Autodesk Inventor part; units mm, degrees
ref_plane "YZ Plane" through (0, 0, 0) normal (1, 0, 0) x (0, 1, 0)
ref_plane "XZ Plane" through (0, 0, 0) normal (0, 1, 0) x (-1, 0, 0)
ref_plane "XY Plane" through (0, 0, 0) normal (0, 0, 1) x (1, 0, 0)
sketch "Sketch1" plane through (0, 0, 0) normal (0, 1, 0) x (-1, 0, 0)
  line L0 (45, 192.5) -> (-45, 192.5)
  line L1 (-45, 192.5) -> (-45, -192.5)
  line L2 (-45, -192.5) -> (45, -192.5)
  line L3 (45, -192.5) -> (45, 192.5)
  line L4 (45, 192.5) -> (-45, -192.5) construction
  line L5 (-45, 192.5) -> (45, -192.5) construction
  line L6 (45, 138.0648) -> (24, 138.0648)
  line L7 (24, 138.0648) -> (24, 113.0648)
  line L8 (24, 113.0648) -> (-11, 113.0648)
  line L9 (-11, 113.0648) -> (-11, 62.0648)
  line L10 (-11, 62.0648) -> (-15.9497, 57.115)
  line L11 (-15.9497, 57.115) -> (-15.9497, -142.885)
  line L12 (-15.9497, -142.885) -> (25.0503, -142.885)
  line L13 (25.0503, -142.885) -> (24, -192.5)
  line L14 (-45, 151.0874) -> (10, 151.0874)
  line L15 (10, 151.0874) -> (10, 180.0874)
  line L16 (10, 180.0874) -> (45, 180.0874)
  line L17 (10, 192.5) -> (-0.6066, 181.8934)
  line L18 (-0.6066, 181.8934) -> (-0.6066, 161.8934)
  line L19 (-0.6066, 161.8934) -> (-35.6066, 161.8934)
  line L20 (-35.6066, 161.8934) -> (-46.4126, 151.0874)
  line L21 (-0.6066, 161.8934) -> (10, 151.0874)
  line L22 (10, 180.0874) -> (3.7937, 186.2937)
  point P0 (0, 0)
  point P1 (-45, 152.5)
  dimension "d0" = 90
  dimension "d1" = 385
  dimension "d25" = 21
  dimension "d27" = 25
  dimension "d28" = 35
  dimension "d29" = 51
  dimension "d30" = 7
  dimension "d31" = 135
  dimension "d32" = 200
  dimension "d33" = 41
  dimension "d34" = 55
  dimension "d35" = 29
  dimension "d36" = 15
  dimension "d37" = 20
  dimension "d38" = 35
extrude "Extrusion1" add sketch "Sketch1" along normal blind 70 contours L3 L16 L22 L17 L0 | L3 L6 L7 L8 L9 L10 L11 L12 L13 L2 L1 L14 L15 L16 | L22 L15 L21 L18 L17 | L20 L19 L21 L14 L1
fillet "Fillet1" radius 20 1 edges at (45, 35, -192.5)
sketch "Sketch2" plane through (0, 70, 0) normal (0, 1, 0) x (1, 0, 0)
  arc A0 (45, 172.5) -> (25, 192.5) centre (25, 172.5) ccw
  line L0 (45, 172.5) -> (25, 172.5)
  line L1 (25, 172.5) -> (25, -161.8934)
  line L2 (0.6066, -161.8934) -> (35.6066, -161.8934)
  line L3 (25, 172.5) -> (25, 192.5171)
  line L4 (25, 192.5171) -> (25, 80.0171)
  line L5 (25, 80.0171) -> (15.9497, 80.0171)
  line L6 (15.9497, 142.885) -> (15.9497, -57.115)
  line L7 (25, 80.0171) -> (25, 5.0171)
  line L8 (25, 5.0171) -> (15.9497, 5.0171)
  line L9 (15.9497, 80.0171) -> (15.9497, 5.0171)
  arc A1 (45, 172.5) -> (25, 192.5) centre (25, 172.5) ccw
  line L10 (25, 192.5) -> (-24, 192.5)
  line L11 (-24, 192.5) -> (-25.0503, 142.885)
  line L12 (-25.0503, 142.885) -> (15.9497, 142.885)
  line L13 (15.9497, 142.885) -> (15.9497, -57.115)
  line L14 (15.9497, -57.115) -> (11, -62.0648)
  line L15 (11, -62.0648) -> (11, -113.0648)
  line L16 (11, -113.0648) -> (-24, -113.0648)
  line L17 (-24, -113.0648) -> (-24, -138.0648)
  line L18 (-24, -138.0648) -> (-45, -138.0648)
  line L19 (-45, -138.0648) -> (-45, -192.5)
  line L20 (45, -152.5) -> (45, 172.5)
  line L21 (25, 5.0171) -> (25, -127.4829)
  line L22 (25, -127.4829) -> (-24, -127.4829)
  line L23 (-45, -192.5) -> (-10, -192.5)
  line L24 (-10, -192.5) -> (0.6066, -181.8934)
  line L25 (0.6066, -181.8934) -> (0.6066, -161.8934)
  line L26 (0.6066, -161.8934) -> (35.6066, -161.8934)
  line L27 (35.6066, -161.8934) -> (45, -152.5)
  point P0 (0, 0)
  dimension "d45" = 112.5
  dimension "d46" = 75
  dimension "d47" = 132.5
extrude "Extrusion2" cut sketch "Sketch2" against normal blind 4 contours L3 L1 L5 L6 L12 L11 L10 | L1 L22 L17 L16 L15 L14 L6 L8
sketch "Sketch3" plane through (0, 0, 0) normal (0, -1, 0) x (1, 0, 0)
  line L0 (25, -192.5) -> (25, -80.0171)
  line L1 (25, -80.0171) -> (15.9497, -80.0171)
  line L2 (15.9497, -5.0171) -> (25, -5.0171)
  line L3 (25, -5.0171) -> (25, 127.4829)
  line L4 (25, 127.4829) -> (-24, 127.4829)
  arc A0 (25, -192.5) -> (45, -172.5) centre (25, -172.5) ccw
  line L5 (45, 152.5) -> (45, -172.5)
  line L6 (35.6066, 161.8934) -> (45, 152.5)
  line L7 (0.6066, 161.8934) -> (35.6066, 161.8934)
  line L8 (0.6066, 181.8934) -> (0.6066, 161.8934)
  line L9 (-10, 192.5) -> (0.6066, 181.8934)
  line L10 (-45, 192.5) -> (-10, 192.5)
  line L11 (-45, 138.0648) -> (-45, 192.5)
  line L12 (-24, 138.0648) -> (-45, 138.0648)
  line L13 (-24, 113.0648) -> (-24, 138.0648)
  line L14 (11, 113.0648) -> (-24, 113.0648)
  line L15 (11, 62.0648) -> (11, 113.0648)
  line L16 (15.9497, 57.115) -> (11, 62.0648)
  line L17 (15.9497, -142.885) -> (15.9497, 57.115)
  line L18 (-25.0503, -142.885) -> (15.9497, -142.885)
  line L19 (-24, -192.5) -> (-25.0503, -142.885)
  line L20 (25, -192.5) -> (-24, -192.5)
  point P0 (0, 0)
extrude "Extrusion3" cut sketch "Sketch3" against normal blind 4 contours L20 L19 L18 L17 L1 L0 | L17 L16 L15 L14 L13 L4 L3 L2
chamfer "Chamfer2" distance 9.3934 angle 45 1 edges at (18.1066, 70, 161.8934)
chamfer "Chamfer3" distance 9.3934 angle 45 2 edges at (0.6066, 70, 171.8934) (-27.5, 70, 192.5)
chamfer "Chamfer4" distance 9.3934 angle 45 1 edges at (18.1066, 0, 161.8934)
chamfer "Chamfer5" distance 9.3934 angle 45 2 edges at (0.6066, 0, 171.8934) (-27.5, 0, 192.5)
sketch "Sketch4" plane through (-45, 0, 138.0648) normal (-1, 0, 0) x (0, 0, 1)
  line L0 (0, 0) -> (0, 70)
  line L1 (0, 0) -> (54.4352, 70)
  line L2 (0, 70) -> (54.4352, 0)
  circle A0 centre (27.2176, 35) radius 18.5
  point P0 (-138.0648, 0)
  dimension "d64" = 37
extrude "Extrusion4" cut sketch "Sketch4" against normal blind 39 contours A0 L2 L1 | L1 L2 A0 | A0 L1 L2 | L1 A0 L2
Can you work these out from the model? Positions are in its coordinate system, mm. A direction names the side the tool comes from. Coordinates: 2 decimals unless noted, no trailing zeros. Loops run counter-clockwise (first coordinate to the right, second up) from the corner with the lowest first, then second, coordinate; pieces in that order, holes last. Notation, with made-up numbers: (1, 43.25) - (46, 43.25) arc R7 cw to (46, 49.25) - close; hole circle Ø5 at (-10, -26.75). An arc over 180 degrees is marked (long way). Answer as a JSON object with one key per item and string values. Group by question number.
Item 1: For pin 1 (2 mm diameter, centred on x = 22.5, y = 1.5, fed in from +Z); pin 2 (2 mm diameter, centred on y = 1.5, z = 64.5, fed in from -X); pin 3 (1.5 mm diameter, centred on x = 13.5, z = -153, fed in from +Y), each with a flat end and sliding along its axis, tell me the tip position at first contact or that it passes through.
Item 2: If we section it at C-C (x = -34): List the corners of the cut face in (y, z) for me.
Item 3: If we section it at B-B (z = -85): List the corners of the cut face in (x, y) for me.
Item 4: On a 3-axis mill with a long thin cutter (end or side, diameter ignored), from which of +Z, -Z, +X, -X, +Y, -Y can I reach the whole of each face in a straight line? I mean faces 4 (the face through (5, 4, -160)), 5 (the face through (-4.156, 4.631, 169.605)), 6 (the face through (-4.156, 65.369, 169.605)). Say none if no direction works.
Item 5: If I drill on L1, parallel to Z at x = -16, y = 35 (3 decimals); L2, parallel to Z at x = -27.5, y = 35; L3, parallel to Z at x = 7.5, y = 40 (3 decimals), over which ranges is the centre line in solid material (lowest first)? Write a range as from..to.
Item 6: If we mould it in two halves opening along Y, with no side actions, what happens to faces 1 (the face through (27, 70, 24)), 2 (the face through (-24, 35, 126)), 3 (the face through (-6, 35, 165))? For each: released by +Y, released by -Y, zero draft, split by the parting line, or undercut.
Item 7: If we section it at A-A (x = 4): List the corners of the cut face in (y, z) for me (3 decimals), plus the area to 3 significant figures.
Item 8: If we section it at D-D (y = 35): List the corners of the cut face in (x, z) for me (3 decimals), plus the area to 3 significant figures.
Returned:
{
 "1": {"pin 1": "stops at z = 155", "pin 2": "stops at x = 25", "pin 3": "stops at y = 66"},
 "2": {"outline": "(0, 138.06) - (70, 138.06) - (70, 183.11) - (60.61, 192.5) - (9.39, 192.5) - (0, 183.11) - close; hole circle Ø37 at (35, 165.28)"},
 "3": {"outline": "(15.95, 4) - (25, 4) - (25, 0) - (45, 0) - (45, 70) - (25, 70) - (25, 66) - (15.95, 66) - close"},
 "4": {"face 4": "-Z, -X, -Y", "face 5": "+Z, +X, -Y", "face 6": "+Z, +X, +Y"},
 "5": {"L1": "z = -192.5..-142.885, 113.065..146.782, 183.782..192.5", "L2": "z = 138.06..146.78, 183.78..192.5", "L3": "z = -192.5..-142.885, 113.065..161.893"},
 "6": {"face 1": "released by +Y", "face 2": "zero draft", "face 3": "undercut"},
 "7": {"outline": "(0, 127.483) - (4, 127.483) - (4, 113.065) - (66, 113.065) - (66, 127.483) - (70, 127.483) - (70, 152.5) - (60.607, 161.893) - (9.393, 161.893) - (0, 152.5) - close; (4, -192.5) - (66, -192.5) - (66, -142.885) - (4, -142.885) - close", "area": "6,290 mm²"},
 "8": {"outline": "(-45, 138.065) - (-24, 138.065) - (-24, 113.065) - (11, 113.065) - (11, 62.065) - (15.95, 57.115) - (15.95, -142.885) - (-25.05, -142.885) - (-24, -192.5) - (25, -192.5) arc R20 ccw to (45, -172.5) - (45, 152.5) - (35.607, 161.893) - (0.607, 161.893) - (0.607, 181.893) - (-10, 192.5) - (-45, 192.5) - (-45, 183.782) - (-6, 183.782) - (-6, 146.782) - (-45, 146.782) - close", "area": "14,800 mm²"}
}
